```python
from build123d import *

# Parameters (mm, degrees)
SKETCH1_R           = 2.5
BOSS_EXTRUDE2_DEPTH = 4


with BuildPart() as part:
    # Sketch1 → Boss-Extrude2 (new body)
    with BuildSketch(Plane(origin=(0, 0, 0), x_dir=(1, 0, 0), z_dir=(0, 1, 0))):
        with BuildLine():
            Line((-20.5, -43.291569618), (-20.5, -11.291569618))
            Line((-20.5, -11.291569618), (20.5, -11.291569618))
            Line((20.5, -11.291569618), (20.5, -43.291569618))
            ThreePointArc((20.5, -43.291569618), (0, 47.9), (-20.5, -43.291569618))
        make_face()
        with Locations(Location((-27.5, 0, 0), (0, 0, 270))):
            Circle(SKETCH1_R, mode=Mode.SUBTRACT)
        with Locations(Location((27.5, 0, 0), (0, 0, 90))):
            Circle(SKETCH1_R, mode=Mode.SUBTRACT)
    extrude(amount=BOSS_EXTRUDE2_DEPTH)


solid = part.part
```
Geometry: final body of the model. Coordinates: model frame, mm. A direction names the side the tool comes from. Coordinates: 2 decimals unless noted, no trailing zeros. Order: outer loops, then holes, each group sorted by start corner. A loop starts at its lowest first (then second) coordinate and runs counter-clockwise, first axis right, second up. Notation, with made-up numbers: (-11, -28.75) - (33, -28.75) arc R15 ccw to (33, -11.75) - close; hole circle Ø10 at (46, 27.25). An arc over 180 degrees is marked (long way). Write each question's results on one line, items separated by ' | '.
1) Set-up query: faces 4 (the cylindrical face through (25, 2, 0)), 5 (the flat face through (20.5, 2, 27)). Return all of +Z, -Z, +X, -X, +Y, -Y with unobstructed straight access to the full face (end or side cutting, diameter ignored); none if empty.
Results list:
face 4: +Y, -Y | face 5: +Z, +Y, -Y
2) Pin query (flat end, axial travel): pin 1 (1 mm diameter, centred on x = 7, y = 3.5, fed in from -Z); pin 2 (2 mm diameter, centred on y = 1.5, z = 27.5, fed in from +X); pin 3 (1 mm diameter, centred on y = 3.5, z = 6.5, fed in from +X). Return the tip coordinate at first contact, or that it passes through.
Results list:
pin 1: z = -47.46 | pin 2: x = 39.9 | pin 3: x = 47.52
3) Pull-direction query (X, two-part tool) for faces 1 (the cylindrical face through (1.81, 1.972, -47.866)), 2 (the flat face through (-1, 0, -3)), 3 (the cylindrical face through (-25, 2, 0)); classes: pulls with the +X half, pulls with the -X half, needs draft (parallel to the pull), parting line crosses it, or undercut.
Results list:
face 1: parting line crosses it | face 2: needs draft | face 3: undercut
4) Section D-D, the plane y = 3. Return loops of the section in (x, z), plus the area to 3 significant figures.
Results list:
outline: (-20.5, 11.29) - (-20.5, 43.29) arc R47.9 ccw (long way) to (20.5, 43.29) - (20.5, 11.29) - close; hole circle Ø5 at (-27.5, 0); hole circle Ø5 at (27.5, 0) | area: 5,730 mm^2
5) Line query: line 1 (X direction, y = 1.7, z = 0); line 2 (X direction, y = 1.75, z = 25); line 3 (Z direction, x = 29, y = 1.3). Output: solid intervals per line, ascending. Write a range as from..to.
Results list:
line 1: -47.9..-30, -25..25, 30..47.9 | line 2: -40.86..-20.5, 20.5..40.86 | line 3: -38.12..-2, 2..38.12
6) Section A-A, the plane z = 0. Return loops of the section in (x, y), plus the area to 3 significant figures.
Results list:
outline: (-47.9, 0) - (-30, 0) - (-30, 4) - (-47.9, 4) - close; (-25, 0) - (25, 0) - (25, 4) - (-25, 4) - close; (30, 0) - (47.9, 0) - (47.9, 4) - (30, 4) - close | area: 343 mm^2
7) Section B-B, the plane x = -27.5. Return loops of the section in (y, z).
Results list:
outline: (0, -39.22) - (4, -39.22) - (4, -2.5) - (0, -2.5) - close; (0, 2.5) - (4, 2.5) - (4, 39.22) - (0, 39.22) - close
8) Section C-C, the plane z = 30. Return loops of the section in (x, y).
Results list:
outline: (-37.34, 0) - (-20.5, 0) - (-20.5, 4) - (-37.34, 4) - close; (20.5, 0) - (37.34, 0) - (37.34, 4) - (20.5, 4) - close
